Geometry check sheet. Reference: the model listing, model coordinates, mm. A direction names the side the tool comes from. Round coordinates to 2 decimals unless told otherwise and drop trailing zeros. Order: outer loops, then holes, each group sorted by start corner. A loop starts at its lowest first (then second) coordinate and runs counter-clockwise, first axis right, second up.
(1) Sectioned sample at D-D (y = 16.25). Record the boundary of the cut face in (x, z).
(2) Sectioned sample at C-C (z = -1). Record the boundary of the cut face in (x, y), plus the area to 3 significant figures.
(3) Go/stop test with flat-tipped pins: pin 1 (3.5 mm diameter, centred on x = -17.93, z = 9, fed in from +Y); pin 2 (1.5 mm diameter, centred on y = 3, z = 5, fed in from +X); pin 3 (11 mm diameter, centred on x = 7, y = 7, fed in from -Z); pin 4 (10 mm diameter, centred on y = 19.5, z = -16.5, fed in from -X). Record where each tip stops, or that it passes through.
(4) Material ranges on line 1 along X through (y, z) = (0.85, 9); line 2 along Y through (x, z) = (-22, -18), recorded low to high.
(5) Release check for a two-part mould opening along Z. For faces 1 (the face through (6, 11, 0)), 2 (the face through (-6, 2, 8)), 3 (the face through (-17.9, 1, 7.4)) record: +Z half, -Z half, draft (parallel to the pull), parting line (faces both ways), or undercut.
(6) Sectioned sample at B-B (x = 0.5). Record the boundary of the cut face in (y, z), plus the area to 3 significant figures.
(7) Set-up check for faces 4 (the face through (-10.929, 13, -12)), 5 (the face through (5, 13, 2)), 6 (the face through (-8.929, 11, -12)): record each of +Z, -Z, +X, -X, +Y, -Y from which the full face is reachable in a straight line by a thin tool's end or side.
(8) Sectioned sample at A-A (z = -15). Record the boundary of the cut face in (x, y), plus the area to 3 significant figures.
from build123d import *

# Parameters (mm, degrees)
BOSS_EXTRUDE1_DEPTH = 2
BOSS_EXTRUDE2_DEPTH = 20
FILLET1_R           = 2
FILLET2_R           = 10
SKETCH3_R           = 1.6
CUT_EXTRUDE1_DEPTH  = 20


with BuildPart() as part:
    # Sketch1 → Boss-Extrude1 (new body)
    with BuildSketch(Plane(origin=(0, 0, 0), x_dir=(1, 0, 0), z_dir=(0, 1, 0))):
        Polygon((-23.929292929, 25), (-8.929292929, 25), (-8.929292929, 0), (21.070707071, 0), (21.070707071, -15), (-23.929292929, -15), align=None)
    extrude(amount=BOSS_EXTRUDE1_DEPTH)

    # Sketch2 → Boss-Extrude2 (add)
    with BuildSketch(Plane(origin=(0, 2, 0), x_dir=(1, 0, 0), z_dir=(0, 1, 0))):
        Polygon((-8.929292929, 25), (-10.929292929, 25), (-10.929292929, -2), (21.070707071, -2), (21.070707071, 0), (-8.929292929, 0), align=None)
    extrude(amount=BOSS_EXTRUDE2_DEPTH)

    # Fillet1
    fillet1_edges = [part.edges().sort_by_distance(p)[0] for p in [
        (-10.929292929, 2, -11.5),
        (5.070707071, 2, 2),
    ]]
    fillet(fillet1_edges, radius=FILLET1_R)

    # Fillet2
    fillet2_edges = [part.edges().sort_by_distance(p)[0] for p in [
        (-23.929292929, 1, 15),
    ]]
    fillet(fillet2_edges, radius=FILLET2_R)

    # Sketch3 → Cut-Extrude1 (cut)
    with BuildSketch(Plane(origin=(0, 2, 0), x_dir=(1, 0, 0), z_dir=(0, 1, 0))):
        with Locations(Location((-17.929292929, 15, 0), (0, 0, 270))):
            Circle(SKETCH3_R)
        with Locations(Location((11.070707071, -9, 0), (0, 0, 270))):
            Circle(SKETCH3_R)
        with Locations(Location((-17.929292929, -9, 0), (0, 0, 270))):
            Circle(SKETCH3_R)
    extrude(amount=-CUT_EXTRUDE1_DEPTH, mode=Mode.SUBTRACT)


solid = part.part
Answer below:
1. outline: (-10.93, -25) - (-8.93, -25) - (-8.93, 0) - (21.07, 0) - (21.07, 2) - (-10.93, 2) - close
2. outline: (-23.93, 0) - (-8.93, 0) - (-8.93, 22) - (-10.93, 22) - (-10.93, 4) arc R2 cw to (-12.93, 2) - (-23.93, 2) - close
2. area: 70.9 mm2
3. pin 1: stops at y = 2
3. pin 2: passes through
3. pin 3: stops at z = 0
3. pin 4: stops at x = -10.93
4. line 1: x = -23.09 to -19.53, -16.33 to 9.47, 12.67 to 21.07
4. line 2: y = 0 to 2
5. face 1: -Z half
5. face 2: draft
5. face 3: undercut
6. outline: (0, 0) - (22, 0) - (22, 2) - (4, 2) arc R2 cw to (2, 4) - (2, 15) - (0, 15) - close
6. area: 70.9 mm2
7. face 4: +Z, -Z, -X, +Y
7. face 5: +Z, +X, -X, +Y
7. face 6: -Z, +X, +Y, -Y
8. outline: (-23.93, 0) - (-19.53, 0) - (-19.53, 2) - (-23.93, 2) - close; (-16.33, 0) - (-8.93, 0) - (-8.93, 22) - (-10.93, 22) - (-10.93, 4) arc R2 cw to (-12.93, 2) - (-16.33, 2) - close
8. area: 64.5 mm2
